```python
from build123d import *

# Parameters (mm, degrees)
F0_W     = 1066.8
F0_H     = 2108.2
F0_W_2   = 76.2
F0_H_2   = 927.1
F1_DEPTH = 22.225
F0_W_3   = 812.8
F0_H_3   = 698.5
F2_DEPTH = 9.525


with BuildPart() as f1:
    # F0 (on Front) → F1 (new body, symmetric)
    with BuildSketch(Plane.XZ):
        Rectangle(F0_W, F0_H)
        Polygon((-406.4, 0), (-406.4, 927.1), (-38.1, 927.1), (38.1, 927.1), (406.4, 927.1), (406.4, 0), (406.4, -127), (406.4, -825.5), (-406.4, -825.5), (-406.4, -127), align=None, mode=Mode.SUBTRACT)
        with Locations((0, 463.55)):
            Rectangle(F0_W_2, F0_H_2)
        Polygon((-38.1, 0), (-406.4, 0), (-406.4, -127), (406.4, -127), (406.4, 0), (38.1, 0), align=None)
    extrude(amount=F1_DEPTH, both=True)

    # F0 (on Front) → F2 (join, symmetric)
    with BuildSketch(Plane.XZ):
        with Locations((0, -476.25)):
            Rectangle(F0_W_3, F0_H_3)
    extrude(amount=F2_DEPTH, both=True)


solid = f1.part
```
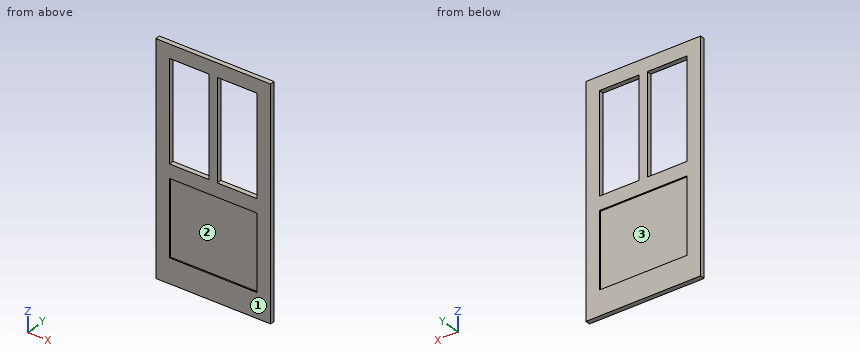
Here's how the part is built. I have some questions about the finished solid (model axes, mm). Face numbers are marked on the shaded views. Give positions to 0.01 mm unless a question says otherwise; leave off trailing zeros. Write each loop counter-clockwise with the first axis right and the second up, starting at its lowest first coordinate (ties: lowest second). Pieces come first, ordered by that corner, then holes. Notation, with made-up numbers: (-18.5, 76.25) -> (26.5, 76.25) arc R25 cw to (26.5, 112.25) -> close; hole circle Ø8 at (67.5, -20). An arc over 180 degrees is marked (long way). Use one line per item in the form item = value.
1) Suppose I cut it at C-C (x = 14.5). Please give me the cut outline in (y, z) (3 decimals).
Verdict:
outline = (-22.225, -1054.1) -> (22.225, -1054.1) -> (22.225, -825.5) -> (9.525, -825.5) -> (9.525, -127) -> (22.225, -127) -> (22.225, 1054.1) -> (-22.225, 1054.1) -> (-22.225, -127) -> (-9.525, -127) -> (-9.525, -825.5) -> (-22.225, -825.5) -> close
2) If I drill on L1, parallel to X at y = -0.5, z = 283; L2, parallel to Z at x = 279, y = 19.5; L3, parallel to Z at x = -180, y = 0.5, over which ranges is the centre line in solid material (lowest first)? Write a range as [from, to].
Verdict:
L1 = [-533.4, -406.4], [-38.1, 38.1], [406.4, 533.4]
L2 = [-1054.1, -825.5], [-127, 0], [927.1, 1054.1]
L3 = [-1054.1, 0], [927.1, 1054.1]
3) I'm going to push a flat-ended pin straight in: pin 1 (2 mm diameter, centred on x = -314.5, z = -688, fed in from +Y) (3 decimals). Where does the tip first touch, or does it pass through?
Verdict:
pin_1 = 9.525
4) Suppose I cut it at B-B (z = 102). Please give me the cut outline in (x, y) (3 decimals).
Verdict:
outline = (-533.4, -22.225) -> (-406.4, -22.225) -> (-406.4, 22.225) -> (-533.4, 22.225) -> close; (-38.1, -22.225) -> (38.1, -22.225) -> (38.1, 22.225) -> (-38.1, 22.225) -> close; (406.4, -22.225) -> (533.4, -22.225) -> (533.4, 22.225) -> (406.4, 22.225) -> close
5) We'd pull the mould along X, two halves only. Please class the marked faces 1, 2 and 3: +X half, -X half, draft (parallel to the pull), parting line (faces both ways), or undercut.
Verdict:
face_1 = draft
face_2 = undercut
face_3 = undercut
6) Suppose I cut it at A-A (x = -262). Please give me the cut outline in (y, z) (3 decimals).
Verdict:
outline = (-22.225, -1054.1) -> (22.225, -1054.1) -> (22.225, -825.5) -> (9.525, -825.5) -> (9.525, -127) -> (22.225, -127) -> (22.225, 0) -> (-22.225, 0) -> (-22.225, -127) -> (-9.525, -127) -> (-9.525, -825.5) -> (-22.225, -825.5) -> close; (-22.225, 927.1) -> (22.225, 927.1) -> (22.225, 1054.1) -> (-22.225, 1054.1) -> close
